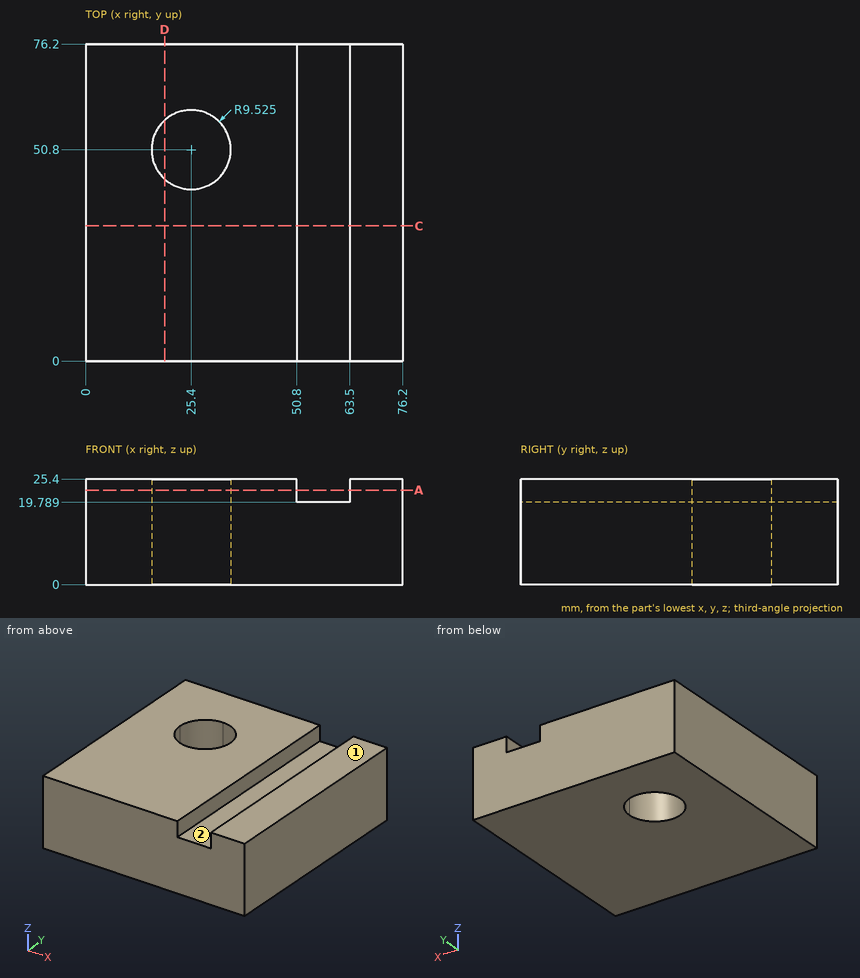
Design review of the part shown in the three views and the two pictorial views. Dimensions are in mm from the part's minimum x, y and z. A direction names the side the tool comes from. Round coordinates to 2 decimals unless told otherwise and drop trailing zeros. Write each loop counter-clockwise with the first axis right and the second up, starting at its lowest first coordinate (ties: lowest second). Pieces come first, ordered by that corner, then holes. Notation, with made-up numbers: (27.5, 80) -> (68.5, 80) arc R25 ccw to (68.5, 115) -> close; hole circle Ø3 at (76.25, -15.75). An arc over 180 degrees is marked (long way). One line per question, with ' | ' between items. Start each with the question number.
1) Add section A-A (z = 22.75). Count the separate pieces of the cut face and the enclosed holes in it, and give its area (3 significant figures).
2) Add section D-D (x = 19). Write out the cut boundary in (y, z) (1 decimal), and give its area (3 significant figures).
3) Add section C-C (y = 32.5). Write out the cut boundary in (x, z).
4) Wall thickness on line 1 along X through (y, z) = (24, 22); line 2 along Y through (x, z) = (31.5, 4.5) (1 decimal); line 3 along Z through (x, y) = (55.5, 43.5): over which ranges is each line inside the solid? List them lowest first.
5) Machinability: for the marked faces 1 and 2, which of the approach directions +Z, -Z, +X, -X, +Y, -Y give a long, thin tool a straight path to every point of the face, cutting with its end or side? Answer none if there is none.
Reported:
1) separate pieces: 2 | enclosed holes: 1 | area: 4,550 mm²
2) outline: (0, 0) -> (43.7, 0) -> (43.7, 25.4) -> (0, 25.4) -> close; (57.9, 0) -> (76.2, 0) -> (76.2, 25.4) -> (57.9, 25.4) -> close | area: 1,580 mm²
3) outline: (0, 0) -> (76.2, 0) -> (76.2, 25.4) -> (63.5, 25.4) -> (63.5, 19.79) -> (50.8, 19.79) -> (50.8, 25.4) -> (0, 25.4) -> close
4) line 1: x = 0 to 50.8, 63.5 to 76.2 | line 2: y = 0 to 43.5, 58.1 to 76.2 | line 3: z = 0 to 19.79
5) face 1: +Z, +X, -X, +Y, -Y | face 2: +Z, +Y, -Y
